Work out the finished part from the listing and answer in its coordinate system (mm). A direction names the side the tool comes from. Coordinates: 2 decimals unless noted, no trailing zeros. Loops run counter-clockwise (first coordinate to the right, second up) from the corner with the lowest first, then second, coordinate; pieces in that order, holes last. Notation, with made-up numbers: (35, -20) -> (49, -20) arc R30 cw to (49, 2) -> close; hole circle Ø6 at (16.25, -37.75). An arc over 180 degrees is marked (long way). One line per question, with ' | ' between items.
```python
from build123d import *

# Parameters (mm, degrees)
SKETCH1_W           = 40.6
SKETCH1_H           = 19.9
BOSS_EXTRUDE1_DEPTH = 27.5
SKETCH2_W           = 54.2
SKETCH2_H           = 19.9
SKETCH2_R           = 2
BOSS_EXTRUDE2_DEPTH = 2.6
SKETCH3_W           = 40.4
SKETCH3_H           = 19.9
BOSS_EXTRUDE3_DEPTH = 6
SKETCH4_R           = 9.95
BOSS_EXTRUDE4_DEPTH = 2
SKETCH5_R           = 6.5
BOSS_EXTRUDE5_DEPTH = 1.5
SKETCH6_R           = 2.85
BOSS_EXTRUDE6_DEPTH = 4.2


with BuildPart() as part:
    # Sketch1 → Boss-Extrude1 (new body)
    with BuildSketch(Plane(origin=(0, 0, 0), x_dir=(1, 0, 0), z_dir=(0, 1, 0))):
        Rectangle(SKETCH1_W, SKETCH1_H)
    extrude(amount=BOSS_EXTRUDE1_DEPTH)

    # Sketch2 → Boss-Extrude2 (add)
    with BuildSketch(Plane(origin=(0, 27.5, 0), x_dir=(1, 0, 0), z_dir=(0, 1, 0))):
        Rectangle(SKETCH2_W, SKETCH2_H)
        with Locations((-24, 4.75)):
            Circle(SKETCH2_R, mode=Mode.SUBTRACT)
        with Locations((-24, -4.75)):
            Circle(SKETCH2_R, mode=Mode.SUBTRACT)
        with Locations((24, -4.75)):
            Circle(SKETCH2_R, mode=Mode.SUBTRACT)
        with Locations((24, 4.75)):
            Circle(SKETCH2_R, mode=Mode.SUBTRACT)
    extrude(amount=BOSS_EXTRUDE2_DEPTH)

    # Sketch3 → Boss-Extrude3 (add)
    with BuildSketch(Plane(origin=(0, 30.1, 0), x_dir=(1, 0, 0), z_dir=(0, 1, 0))):
        Rectangle(SKETCH3_W, SKETCH3_H)
    extrude(amount=BOSS_EXTRUDE3_DEPTH)

    # Sketch4 → Boss-Extrude4 (add)
    with BuildSketch(Plane(origin=(0, 36.1, 0), x_dir=(1, 0, 0), z_dir=(0, 1, 0))):
        with BuildLine():
            Line((14.2, 9.95), (-10.25, 9.95))
            ThreePointArc((-10.25, 9.95), (-3.214287527, 7.035712473), (-0.3, 0))
            ThreePointArc((-0.3, 0), (-3.214287527, -7.035712473), (-10.25, -9.95))
            Line((-10.25, -9.95), (14.2, -9.95))
            Line((14.2, -9.95), (14.2, 9.95))
        make_face()
        with Locations((-10.25, 0)):
            Circle(SKETCH4_R)
    extrude(amount=BOSS_EXTRUDE4_DEPTH)

    # Sketch5 → Boss-Extrude5 (add)
    with BuildSketch(Plane(origin=(0, 38.1, 0), x_dir=(1, 0, 0), z_dir=(0, 1, 0))):
        with Locations((-10.25, 0)):
            Circle(SKETCH5_R)
    extrude(amount=BOSS_EXTRUDE5_DEPTH)

    # Sketch6 → Boss-Extrude6 (add)
    with BuildSketch(Plane(origin=(0, 39.6, 0), x_dir=(1, 0, 0), z_dir=(0, 1, 0))):
        with Locations((-10.25, 0)):
            Circle(SKETCH6_R)
    extrude(amount=BOSS_EXTRUDE6_DEPTH)


solid = part.part
```
1) Find section C-C (y = 41). Write down the section's boundary in (x, z), plus the area to 3 significant figures.
Check values:
outline: circle Ø5.7 at (-10.25, 0) | area: 25.5 mm^2
2) For faces 4 (the face through (14.2, 37, 0)), 5 (the face through (-24, 27.5, 0)), 6 (the face through (-4.05, 38.84, -1.95)), 7 (the face through (20.3, 14, 0)), 8 (the face through (-18, 36.1, 8)), determine the directions among +Z, -Z, +X, -X, +Y, -Y from which every point of the face is accessible in a straight line to the end or side of a thin tool.
Check values:
face 4: +Z, -Z, +X, +Y | face 5: +Z, -Z, -X, -Y | face 6: +Y | face 7: +Z, -Z, +X, -Y | face 8: +Z, -X, +Y
3) Find the intervals of material crossed by line 1 along Z through (x, y) = (24, 28.4); line 2 along X through (y, z) = (28.85, 4.75); line 3 along X through (y, z) = (13, 7), in increasing order.
Check values:
line 1: z = -9.95 to -6.75, -2.75 to 2.75, 6.75 to 9.95 | line 2: x = -27.1 to -26, -22 to 22, 26 to 27.1 | line 3: x = -20.3 to 20.3
4) Find section B-B (x = 24). Write down the section's boundary in (y, z).
Check values:
outline: (27.5, -9.95) -> (30.1, -9.95) -> (30.1, -6.75) -> (27.5, -6.75) -> close; (27.5, -2.75) -> (30.1, -2.75) -> (30.1, 2.75) -> (27.5, 2.75) -> close; (27.5, 6.75) -> (30.1, 6.75) -> (30.1, 9.95) -> (27.5, 9.95) -> close
5) Flat-ended cylindrical pins translate along their axes: pin 1 (6 mm diameter, centred on y = 8, z = -2.5, fed in from -X); pin 2 (8 mm diameter, centred on x = -17, z = -4.5, fed in from +Y); pin 3 (3.5 mm diameter, centred on x = 22.5, z = -4, fed in from -Y). Find the tip coordinate at first contact, or state that the pin passes through.
Check values:
pin 1: stops at x = -20.3 | pin 2: stops at y = 39.6 | pin 3: stops at y = 27.5
6) Find section D-D (x = -16). Write down the section's boundary in (y, z).
Check values:
outline: (0, -9.95) -> (36.1, -9.95) -> (36.1, -8.12) -> (38.1, -8.12) -> (38.1, -3.03) -> (39.6, -3.03) -> (39.6, 3.03) -> (38.1, 3.03) -> (38.1, 8.12) -> (36.1, 8.12) -> (36.1, 9.95) -> (0, 9.95) -> close
7) Find section A-A (z = 5.5). Write down the section's boundary in (x, y).
Check values:
outline: (-27.1, 27.5) -> (-25.85, 27.5) -> (-25.85, 30.1) -> (-27.1, 30.1) -> close; (-22.15, 27.5) -> (-20.3, 27.5) -> (-20.3, 0) -> (20.3, 0) -> (20.3, 27.5) -> (22.15, 27.5) -> (22.15, 30.1) -> (20.2, 30.1) -> (20.2, 36.1) -> (14.2, 36.1) -> (14.2, 38.1) -> (-6.79, 38.1) -> (-6.79, 39.6) -> (-13.71, 39.6) -> (-13.71, 38.1) -> (-18.54, 38.1) -> (-18.54, 36.1) -> (-20.2, 36.1) -> (-20.2, 30.1) -> (-22.15, 30.1) -> close; (25.85, 27.5) -> (27.1, 27.5) -> (27.1, 30.1) -> (25.85, 30.1) -> close
8) The mould has two halves that part along X. Classify faces 1 (the face through (22.413, 28.782, 5.967)), 2 (the face through (-27.1, 29, 0)), 3 (the face through (-7, 39.6, 1)): released by +X, released by -X, zero draft, split by the parting line, or undercut.
Check values:
face 1: undercut | face 2: released by -X | face 3: zero draft
